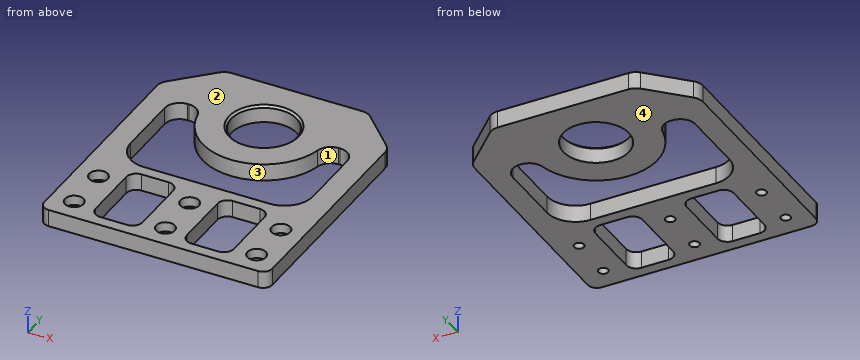
```python
from build123d import *

# Parameters (mm, degrees)
SKETCH1_W                                           = 80
SKETCH1_H                                           = 115
BOSS_EXTRUDE1_DEPTH                                 = 6
CBORE_FOR_M3_HEX_SOCKET_HEAD_CAP_SCREW1_D           = 3.4
CBORE_FOR_M3_HEX_SOCKET_HEAD_CAP_SCREW1_CBORE_D     = 6.5
CBORE_FOR_M3_HEX_SOCKET_HEAD_CAP_SCREW1_CBORE_DEPTH = 3.4
SKETCH4_R                                           = 11.5
CUT_EXTRUDE1_DEPTH                                  = 141.2176879
CHAMFER1_SIZE                                       = 0.75
CHAMFER2_SIZE                                       = 6
CBORE_START                                         = 2.6
CBORE_FOR_M3_HEX_SOCKET_HEAD_CAP_SCR_2_R            = 3.25
CBORE_FOR_M3_HEX_SOCKET_HEAD_CAP_SCREW2_DEPTH       = 3.4
CBORE_FOR_M3_HEX_SOCKET_HEAD_CAP_SCR_3_O_R          = 1.7
CBORE_FOR_M3_HEX_SOCKET_HEAD_CAP_SCR_3_DEPTH        = 2.6
CUT_EXTRUDE2_DEPTH                                  = 141.2176879
FILLET1_R                                           = 3.25
CUT_EXTRUDE3_DEPTH                                  = 141.2176879
FILLET2_R                                           = 10
FILLET4_R                                           = 5.25
SKETCH10_W                                          = 16.5
SKETCH10_H                                          = 27.25
CUT_EXTRUDE4_DEPTH                                  = 141.2176879
FILLET5_R                                           = 3.5
SKETCH11_W                                          = 80
SKETCH11_H                                          = 20.198039027
CUT_EXTRUDE5_DEPTH                                  = 141.2176879
CHAMFER3_SIZE                                       = 15
FILLET6_R                                           = 5


# Read off the part's stored shape, not the designer's step: CBORE for M3 Hex Socket Head Cap Screw2
with BuildPart() as part:
    # Sketch1 → Boss-Extrude1 (new body)
    with BuildSketch(Plane.XY):
        with Locations((40, 57.5)):
            Rectangle(SKETCH1_W, SKETCH1_H)
    extrude(amount=BOSS_EXTRUDE1_DEPTH)

    # CBORE for M3 Hex Socket Head Cap Screw1 (through all)
    with Locations(Plane.XY.offset(6)):
        with Locations((8, 8), (40, 8), (72, 8), (40, 24), (72, 24), (8, 24)):
            CounterBoreHole(CBORE_FOR_M3_HEX_SOCKET_HEAD_CAP_SCREW1_D / 2, CBORE_FOR_M3_HEX_SOCKET_HEAD_CAP_SCREW1_CBORE_D / 2, CBORE_FOR_M3_HEX_SOCKET_HEAD_CAP_SCREW1_CBORE_DEPTH)

    # Sketch4 → Cut-Extrude1 (cut, through all)
    with BuildSketch(Plane.XY.offset(6)):
        with Locations((40, 73)):
            Circle(SKETCH4_R)
    extrude(amount=-CUT_EXTRUDE1_DEPTH, mode=Mode.SUBTRACT)

    # Chamfer1
    chamfer1_edges = [part.edges().sort_by_distance(p)[0] for p in [
        (28.5, 73, 6),
    ]]
    chamfer(chamfer1_edges, length=CHAMFER1_SIZE)

    # Chamfer2
    chamfer2_edges = [part.edges().sort_by_distance(p)[0] for p in [
        (0, 115, 3),
        (80, 115, 3),
    ]]
    chamfer(chamfer2_edges, length=CHAMFER2_SIZE)

    # CBORE for M3 Hex Socket Head Cap Scr 2 → CBORE for M3 Hex Socket Head Cap Screw2 (cut)
    with BuildSketch(Plane.XY.offset(CBORE_START)):
        with Locations((8, 105)):
            Circle(CBORE_FOR_M3_HEX_SOCKET_HEAD_CAP_SCR_2_R)
        with Locations((72, 105)):
            Circle(CBORE_FOR_M3_HEX_SOCKET_HEAD_CAP_SCR_2_R)
    extrude(amount=CBORE_FOR_M3_HEX_SOCKET_HEAD_CAP_SCREW2_DEPTH, mode=Mode.SUBTRACT)

    # CBORE for M3 Hex Socket Head Cap Scr 3 o → CBORE for M3 Hex Socket Head Cap Scr 3 (cut)
    with BuildSketch(Plane.XY):
        with Locations((8, 105)):
            Circle(CBORE_FOR_M3_HEX_SOCKET_HEAD_CAP_SCR_3_O_R)
        with Locations((72, 105)):
            Circle(CBORE_FOR_M3_HEX_SOCKET_HEAD_CAP_SCR_3_O_R)
    extrude(amount=CBORE_FOR_M3_HEX_SOCKET_HEAD_CAP_SCR_3_DEPTH, mode=Mode.SUBTRACT)

    # Sketch8 → Cut-Extrude2 (cut, through all)
    with BuildSketch(Plane.XY.offset(6)):
        Polygon((18.198039027, 105), (18.198039027, 94.801960973), (40, 94.801960973), (61.801960973, 94.801960973), (61.801960973, 105), (61.801960973, 115), (18.198039027, 115), align=None)
    extrude(amount=-CUT_EXTRUDE2_DEPTH, mode=Mode.SUBTRACT)

    # Fillet1
    fillet1_edges = [part.edges().sort_by_distance(p)[0] for p in [
        (61.801960973, 115, 3),
        (61.801960973, 94.801960973, 3),
        (18.198039027, 94.801960973, 3),
        (18.198039027, 115, 3),
        (0, 109, 3),
        (74, 115, 3),
        (6, 115, 3),
        (80, 109, 3),
        (80, 0, 3),
        (0, 0, 3),
    ]]
    fillet(fillet1_edges, radius=FILLET1_R)

    # Sketch9 → Cut-Extrude3 (cut, through all)
    with BuildSketch(Plane.XY.offset(6)):
        with BuildLine():
            Line((8, 73), (8, 35.25))
            Line((8, 35.25), (40, 35.25))
            Line((40, 35.25), (72, 35.25))
            Line((72, 35.25), (72, 73))
            Line((72, 73), (61.5, 73))
            ThreePointArc((61.5, 73), (40, 51.5), (18.5, 73))
            Line((18.5, 73), (8, 73))
        make_face()
    extrude(amount=-CUT_EXTRUDE3_DEPTH, mode=Mode.SUBTRACT)

    # Fillet2
    fillet2_edges = [part.edges().sort_by_distance(p)[0] for p in [
        (72, 35.25, 3),
        (8, 35.25, 3),
    ]]
    fillet(fillet2_edges, radius=FILLET2_R)

    # Fillet4
    fillet4_edges = [part.edges().sort_by_distance(p)[0] for p in [
        (18.5, 73, 3),
        (61.5, 73, 3),
        (72, 73, 3),
        (8, 73, 3),
    ]]
    fillet(fillet4_edges, radius=FILLET4_R)

    # Sketch10 → Cut-Extrude4 (cut, through all)
    with BuildSketch(Plane.XY.offset(6)):
        with Locations((24, 17.625)):
            Rectangle(SKETCH10_W, SKETCH10_H)
        with Locations((56, 17.625)):
            Rectangle(SKETCH10_W, SKETCH10_H)
    extrude(amount=-CUT_EXTRUDE4_DEPTH, mode=Mode.SUBTRACT)

    # Fillet5
    fillet5_edges = [part.edges().sort_by_distance(p)[0] for p in [
        (15.75, 31.25, 3),
        (32.25, 31.25, 3),
        (32.25, 4, 3),
        (15.75, 4, 3),
        (47.75, 31.25, 3),
        (64.25, 31.25, 3),
        (64.25, 4, 3),
        (47.75, 4, 3),
    ]]
    fillet(fillet5_edges, radius=FILLET5_R)

    # Sketch11 → Cut-Extrude5 (cut, through all)
    with BuildSketch(Plane.XY.offset(6)):
        with Locations((40, 104.900980487)):
            Rectangle(SKETCH11_W, SKETCH11_H)
    extrude(amount=-CUT_EXTRUDE5_DEPTH, mode=Mode.SUBTRACT)

    # Chamfer3
    chamfer3_edges = [part.edges().sort_by_distance(p)[0] for p in [
        (80, 94.801960973, 3),
        (0, 94.801960973, 3),
    ]]
    chamfer(chamfer3_edges, length=CHAMFER3_SIZE)

    # Fillet6
    fillet6_edges = [part.edges().sort_by_distance(p)[0] for p in [
        (80, 79.801960973, 3),
        (15, 94.801960973, 3),
        (65, 94.801960973, 3),
        (0, 79.801960973, 3),
    ]]
    fillet(fillet6_edges, radius=FILLET6_R)


solid = part.part
```
Can you work these out from the model? Positions are in its coordinate system, mm. Face numbers are marked on the shaded views. A direction names the side the tool comes from. Round coordinates to 2 decimals unless told otherwise and drop trailing zeros.
(1) I'm going to push a flat-ended pin straight in: pin 1 (4 mm diameter, centred on x = 40, y = 24, fed in from +Z). Where does the tip first touch, or does it pass through?
Results are:
pin 1: stops at z = 2.6
(2) On a 3-axis mill with a long thin cutter (end or side, diameter ignored), from which of +Z, -Z, +X, -X, +Y, -Y can I reach the whole of each face in a straight line? I mean the marked faces 3 and 4. Say none if no direction works.
Results are:
face 3: +Z, -Z
face 4: -Z, +X, -X, +Y, -Y
(3) If we section it at A-A (x = 40): Count the separate pieces of the cut face and the enclosed holes in it, plus the area to 3 significant figures.
Results are:
separate pieces: 5
enclosed holes: 0
area: 271 mm2
(4) We'd pull the mould along Y, two halves only. Please class the marked faces 1 and 2: +Y half, -Y half, draft (parallel to the pull), parting line (faces both ways), or undercut.
Results are:
face 1: undercut
face 2: draft
(5) If I drill on L1, parallel to X at y = 20.5, z = 4.75; L2, parallel to X at y = 26.5, z = 5.75; L3, parallel to Y at x = 21, z = 0.5, over which ranges is the centre line in solid material (lowest first)?
Results are:
L1: x = 0 to 15.75, 32.25 to 47.75, 64.25 to 80
L2: x = 0 to 5.92, 10.08 to 15.75, 32.25 to 37.92, 42.08 to 47.75, 64.25 to 69.92, 74.08 to 80
L3: y = 0 to 4, 31.25 to 35.25, 62.94 to 94.8
